Source: CAD feature listing. Evaluate the final solid. Frame: model axes, mm. Face numbers are marked on the shaded views. A direction names the side the tool comes from. Give positions to 0.01 mm unless a question says otherwise; leave off trailing zeros. Order: outer loops, then holes, each group sorted by start corner. A loop starts at its lowest first (then second) coordinate and runs counter-clockwise, first axis right, second up. Notation, with made-up numbers: M 56,70.5 L 94,70.5 A23 cw 94,78.5 Z; hole C 37,46.25 d11. An arc over 180 degrees is marked long. Use CSV: the item, a comma, the result in double quotes. Start each with the question number.
Item 1: Section query B-B on y = 11.5. Return loops of the section in (x, z), and give its area (3 significant figures).
Item 2: Section query D-D on z = 6. Return loops of the section in (x, y), and give its area (3 significant figures).
Item 3: Section query C-C on x = -7. Return loops of the section in (y, z), and give its area (3 significant figures).
Item 4: Pull-direction query (X, two-part tool) for the marked faces 1, 2 and 3; classes: +X half, -X half, draft (parallel to the pull), parting line (faces both ways), or undercut.
Item 5: Ray query, probe 1 along X at (y, z) = (-19, 2.75); probe 2 along X at (y, z) = (-28, -2.5); probe 3 along Y at (x, z) = (-25, 1.25). Return the intervals inside material, ascending. Write a range as from..to.
Item 6: First-contact query: pin 1 (5.5 mm diameter, centred on y = -23.5, z = -1.5, fed in from +X); pin 2 (6 mm diameter, centred on x = -9, z = -1, fed in from +Y); pin 3 (10 mm diameter, centred on x = -2.5, y = -13.5, fed in from +Z); pin 4 (5 mm diameter, centred on x = -3.5, z = 0.5, fed in from -Y). Flat tips, straight axial feed; report the tip coordinate or a pass-through.
Item 7: Access query for the marked faces 4, 5, 6, 7 and 8. Directions: +Z, -Z, +X, -X, +Y, -Y. A direction counts if a zero-diameter tool reaches every point of the face in a straight line with its end or side. Return the directions, or none.
Item 8: Section query A-A on x = -1. Return loops of the section in (y, z).
from build123d import *

# Parameters (mm, degrees)
F1_DEPTH = 27.5
F2_DEPTH = 12.5
F3_DEPTH = 18.5
F4_R     = 3.35
F5_DEPTH = 8.4572335871


with BuildPart() as f1:
    # F0 (on Right) → F1 (new body, symmetric)
    with BuildSketch(Plane.YZ):
        Polygon((2.0231563184, 7.7193960785), (2.0231563184, 0), (14.0231563184, 0), (14.0231563184, 4.9995293425), align=None)
        Polygon((-3.6268436816, 9), (-3.6268436816, 0), (2.0231563184, 0), (2.0231563184, 7.7193960785), align=None)
    extrude(amount=F1_DEPTH, both=True)

    # F0 (on Right) → F2 (join, symmetric)
    with BuildSketch(Plane.YZ):
        Polygon((-15.6079412508, -4.360762889), (-3.6268436816, 0), (-3.6268436816, 9), (-18.5004854943, 3.586437105), align=None)
        Polygon((-27.5890355811, -8.7215245992), (-15.6079412508, -4.360762889), (-18.5004854943, 3.586437105), (-30.4815798247, -0.7743246052), align=None)
    extrude(amount=F2_DEPTH, both=True)

    # F0 (on Right) → F3 (cut, symmetric)
    with BuildSketch(Plane.YZ):
        Polygon((2.0231563184, 7.7193960785), (2.0231563184, 0), (14.0231563184, 0), (14.0231563184, 4.9995293425), align=None)
    extrude(amount=F3_DEPTH, both=True, mode=Mode.SUBTRACT)

    # F4 (on face) → F5 (cut, through all)
    with BuildSketch(Plane(origin=(0, -3.3168043602, 9.1128450844), x_dir=(1, 0, 0), z_dir=(0, -0.3420201433, 0.9396926208))):
        with Locations((0, -16.1581359673)):
            Circle(F4_R)
    extrude(amount=-F5_DEPTH, mode=Mode.SUBTRACT)


solid = f1.part
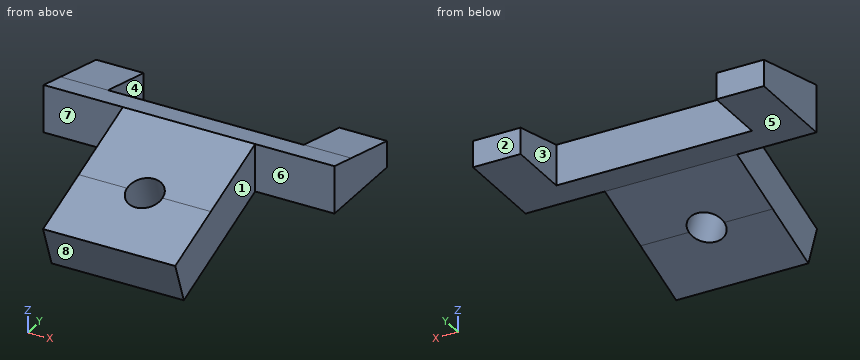
Verdict:
1,outline,"M -27.5,0 L -18.5,0 L -18.5,5.57 L -27.5,5.57 Z; M 18.5,0 L 27.5,0 L 27.5,5.57 L 18.5,5.57 Z"
1,area,"100 mm2"
2,outline,"M -27.5,-3.63 L -12.5,-3.63 L -12.5,-11.87 L 12.5,-11.87 L 12.5,-3.63 L 27.5,-3.63 L 27.5,9.61 L 18.5,9.61 L 18.5,2.02 L -18.5,2.02 L -18.5,9.61 L -27.5,9.61 Z"
2,area,"653 mm2"
3,outline,"M -30.48,-0.77 L -27.59,-8.72 L -3.63,0 L 2.02,0 L 2.02,7.72 L -3.63,9 Z"
3,area,"276 mm2"
4,face 1,"+X half"
4,face 2,"draft"
4,face 3,"undercut"
5,probe 1,"-12.5..-3.26, 3.26..12.5"
5,probe 2,"-12.5..12.5"
5,probe 3,"-3.63..14.02"
6,pin 1,"x = 12.5"
6,pin 2,"y = 2.02"
6,pin 3,"z = 7.23"
6,pin 4,"y = -30.48"
7,face 4,"+Z, -Z, +Y"
7,face 5,"-Z, +X, -X, +Y"
7,face 6,"+Z, -Z, +X, -Y"
7,face 7,"+Z, -Z, -X, -Y"
7,face 8,"-Z, +X, -X, -Y"
8,outline,"M -30.48,-0.77 L -27.59,-8.72 L -18.61,-5.45 L -21.5,2.49 Z; M -15.5,4.68 L -12.6,-3.27 L -3.63,0 L 2.02,0 L 2.02,7.72 L -3.63,9 Z"
